from build123d import *

# Parameters (mm, degrees)
SKETCH_1_W          = 64
SKETCH_1_H          = 64
EXTRUDE_1_DEPTH     = 2
SKETCH_2_R          = 1.6
CUT_EXTRUDE_1_DEPTH = 2
FILLET_1_R          = 4
CUT_EXTRUDE_2_DEPTH = 10
CUT_EXTRUDE_3_DEPTH = 10
FILLET_2_R          = 3
SKETCH_5_R          = 6
CUT_EXTRUDE_4_DEPTH = 10


with BuildPart() as part:
    # 草图1 → 凸台-拉伸1 (new body)
    with BuildSketch(Plane.XY):
        Rectangle(SKETCH_1_W, SKETCH_1_H)
    extrude(amount=EXTRUDE_1_DEPTH)

    # 草图2 → 切除-拉伸1 (cut)
    with BuildSketch(Plane.XY.offset(2)):
        with Locations((-27.5, -27.5)):
            Circle(SKETCH_2_R)
        with Locations((-27.5, 27.5)):
            Circle(SKETCH_2_R)
        with Locations(Location((27.5, -27.5, 0), (0, 0, 180))):
            Circle(SKETCH_2_R)
        with Locations(Location((27.5, 27.5, 0), (0, 0, 180))):
            Circle(SKETCH_2_R)
    extrude(amount=-CUT_EXTRUDE_1_DEPTH, mode=Mode.SUBTRACT)

    # 圆角1
    fillet_1_edges = [part.edges().sort_by_distance(p)[0] for p in [
        (32, -32, 1),
        (-32, -32, 1),
        (-32, 32, 1),
        (32, 32, 1),
    ]]
    fillet(fillet_1_edges, radius=FILLET_1_R)

    # 草图3 → 切除-拉伸2 (cut)
    with BuildSketch(Plane.XY.offset(2)):
        with BuildLine():
            Line((-20.8, 8), (-20.8, -8))
            ThreePointArc((-20.8, -8), (-24, -11.2), (-27.2, -8))
            Line((-27.2, -8), (-27.2, 8))
            ThreePointArc((-27.2, 8), (-24, 11.2), (-20.8, 8))
        make_face()
        with BuildLine():
            Line((20.8, 8), (20.8, -8))
            ThreePointArc((20.8, -8), (24, -11.2), (27.2, -8))
            Line((27.2, -8), (27.2, 8))
            ThreePointArc((27.2, 8), (24, 11.2), (20.8, 8))
        make_face()
    extrude(amount=-CUT_EXTRUDE_2_DEPTH, mode=Mode.SUBTRACT)

    # 草图4 → 切除-拉伸3 (cut)
    with BuildSketch(Plane.XY.offset(2)):
        Polygon((-15.498284962, 22.363155997), (-15.498284962, -22.363155997), (-2.32136638, 0), align=None)
        Polygon((-13.587694119, -27), (13.587694119, -27), (0, -3.939697902), align=None)
        Polygon((2.32136638, 0), (15.498284962, 22.363155997), (15.498284962, -22.363155997), align=None)
        Polygon((0, 3.939697902), (-13.587694119, 27), (13.587694119, 27), align=None)
    extrude(amount=-CUT_EXTRUDE_3_DEPTH, mode=Mode.SUBTRACT)

    # 圆角2
    fillet_2_edges = [part.edges().sort_by_distance(p)[0] for p in [
        (15.498284962, -22.363155997, 1),
        (2.32136638, 0, 1),
        (15.498284962, 22.363155997, 1),
        (-13.587694119, -27, 1),
        (0, -3.939697902, 1),
        (13.587694119, -27, 1),
        (13.587694119, 27, 1),
        (0, 3.939697902, 1),
        (-13.587694119, 27, 1),
        (-2.32136638, 0, 1),
        (-15.498284962, -22.363155997, 1),
        (-15.498284962, 22.363155997, 1),
    ]]
    fillet(fillet_2_edges, radius=FILLET_2_R)

    # 草图5 → 切除-拉伸4 (cut)
    with BuildSketch(Plane.XY.offset(2)):
        with Locations((21, 20)):
            Circle(SKETCH_5_R)
        with Locations((-21, 20)):
            Circle(SKETCH_5_R)
        with Locations((21, -20)):
            Circle(SKETCH_5_R)
        with Locations((-21, -20)):
            Circle(SKETCH_5_R)
    extrude(amount=-CUT_EXTRUDE_4_DEPTH, mode=Mode.SUBTRACT)


solid = part.part
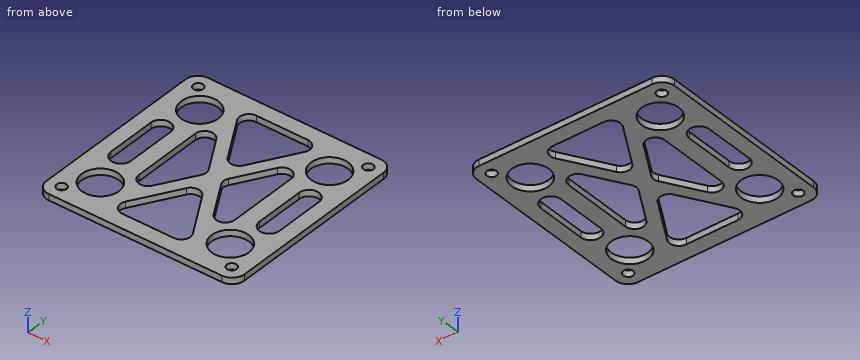
Design review of the part built by this model. Coordinates are the model's own, in mm. Give positions to 0.01 mm unless a question says otherwise; leave off trailing zeros. Loops run counter-clockwise (first coordinate to the right, second up) from the corner with the lowest first, then second, coordinate; pieces in that order, holes last. Notation, with made-up numbers: (6.5, 61) -> (15.5, 61) arc R7 ccw to (15.5, 69) -> close; hole circle Ø8 at (8, -37). An arc over 180 degrees is marked (long way). One line per question, with ' | ' between items. Start each with the question number.
(1) For line 1 (Y direction, x = -27.5, z = 0.6); line 2 (Y direction, x = 6, z = 1.45); line 3 (X direction, y = 14.5, z = 1.35), list the stretches that pass through material, from the lowest coordinate up.
(2) We need section A-A (x = -24). State the section outline as (y, z) points.
(3) We need section D-D (z = 1.35). State how many separate pieces and enclosed holes the cut face has, and give its area (3 significant figures).
(4) We need section B-B (y = -18.5). State the section outline as (x, z) points, and give its area (3 significant figures).
(5) We need section C-C (x = 0). State the section outline as (y, z) points.
The answers:
1) line 1: y = -32 to -29.1, -25.9 to 25.9, 29.1 to 32 | line 2: y = -32 to -27, -14.12 to -6.24, 6.24 to 14.12, 27 to 32 | line 3: x = -32 to -23.4, -18.6 to -6.22, 6.22 to 18.6, 23.4 to 32
2) outline: (-32, 0) -> (-25.2, 0) -> (-25.2, 2) -> (-32, 2) -> close; (-14.8, 0) -> (-11.2, 0) -> (-11.2, 2) -> (-14.8, 2) -> close; (11.2, 0) -> (14.8, 0) -> (14.8, 2) -> (11.2, 2) -> close; (25.2, 0) -> (32, 0) -> (32, 2) -> (25.2, 2) -> close
3) separate pieces: 1 | enclosed holes: 14 | area: 2,240 mm^2
4) outline: (-32, 0) -> (-26.81, 0) -> (-26.81, 2) -> (-32, 2) -> close; (-15.19, 0) -> (-8.58, 0) -> (-8.58, 2) -> (-15.19, 2) -> close; (8.58, 0) -> (15.19, 0) -> (15.19, 2) -> (8.58, 2) -> close; (26.81, 0) -> (32, 0) -> (32, 2) -> (26.81, 2) -> close | area: 47.2 mm^2
5) outline: (-32, 0) -> (-27, 0) -> (-27, 2) -> (-32, 2) -> close; (-6.85, 0) -> (6.85, 0) -> (6.85, 2) -> (-6.85, 2) -> close; (27, 0) -> (32, 0) -> (32, 2) -> (27, 2) -> close
